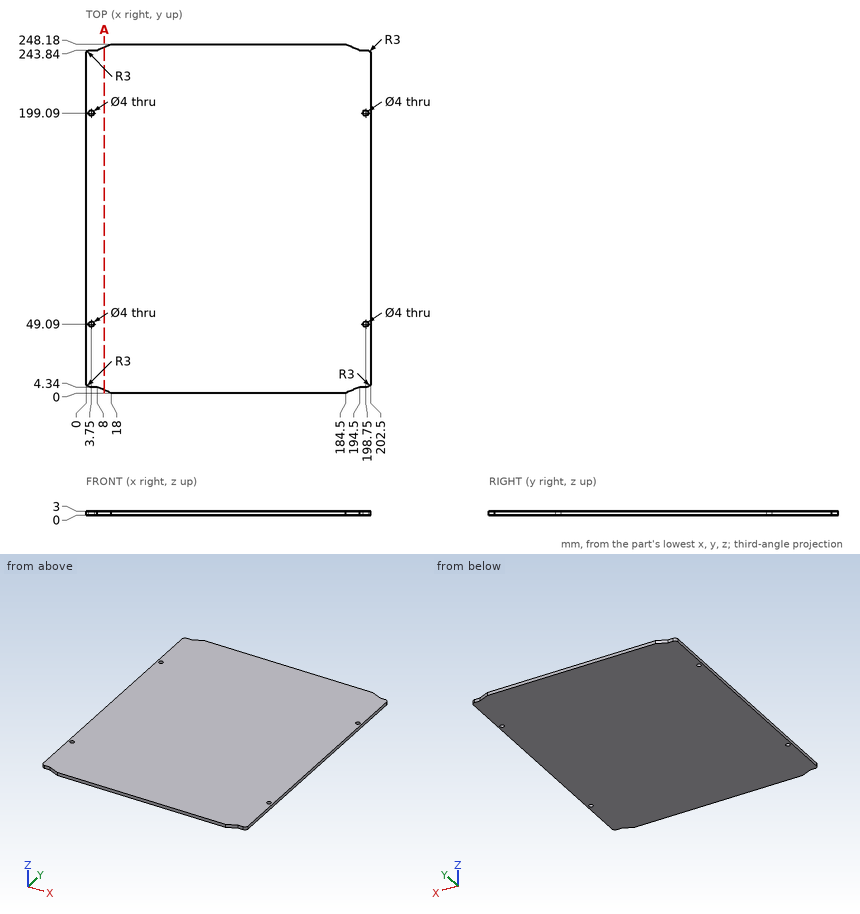
Geometry check sheet. Reference: drawing and pictorial views, mm from the part's lowest x, y, z. Give positions to 0.01 mm unless a question says otherwise; leave off trailing zeros. Loops run counter-clockwise (first coordinate to the right, second up) from the corner with the lowest first, then second, coordinate; pieces in that order, holes last. Notation, with made-up numbers: (11, -9.5) - (32, -9.5) arc R9 cw to (32, -5.5) - close; hole circle Ø10 at (20, 80.25). An arc over 180 degrees is marked (long way). Use CSV: the item, a comma, the result in double quotes. Start each with the question number.
Q1. Scan lines: probe 1 along X at (y, z) = (199.09, 1.5); probe 2 along Y at (x, z) = (3.75, 1.9); probe 3 along X at (y, z) = (50.5, 0.45). Record each from-to range of solid material in increasing order. Write a range as from..to.
Q2. Go/stop test with flat-tipped pins: pin 1 Ø1.5 at (x, z) = (198, 2) entering from -Y; pin 2 Ø0.9 at (x, z) = (197, 1) entering from +Y. Record where each tip stops, or that it passes through.
Q3. Section check A-A, the plane x = 13. Record the cut outline in (y, z).
Findings below:
1,probe 1,"x = 0..1.75, 5.75..196.75, 200.75..202.5"
1,probe 2,"y = 4.34..47.09, 51.09..197.09, 201.09..243.84"
1,probe 3,"x = 0..2.33, 5.17..197.33, 200.17..202.5"
2,pin 1,"stops at y = 4.34"
2,pin 2,"stops at y = 243.84"
3,outline,"(2.17, 0) - (246.01, 0) - (246.01, 3) - (2.17, 3) - close"
